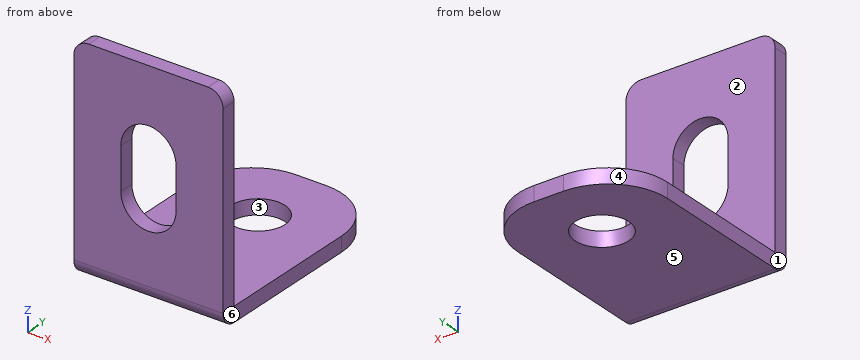
Autodesk Inventor part; units mm, degrees
ref_plane "YZ Plane" through (0, 0, 0) normal (1, 0, 0) x (0, 1, 0)
ref_plane "XZ Plane" through (0, 0, 0) normal (0, 1, 0) x (-1, 0, 0)
ref_plane "XY Plane" through (0, 0, 0) normal (0, 0, 1) x (1, 0, 0)
sketch "Sketch1" plane through (0, 0, 0) normal (0, 1, 0) x (-1, 0, 0)
  line L0 (5, 7.3) -> (-5, 7.3)
  line L1 (-5, 7.3) -> (-5, -7.3)
  line L2 (-5, -7.3) -> (5, -7.3)
  line L3 (5, -7.3) -> (5, 7.3)
  line L4 (5, 7.3) -> (-5, -7.3) construction
  line L5 (-5, 7.3) -> (5, -7.3) construction
  point P0 (0, 0)
  dimension "d0" = 10
  dimension "d1" = 14.6
extrude "Extrusion1" add sketch "Sketch1" along normal blind 1
sketch "Sketch2" plane through (5, 0, -7.3) normal (0, 0, -1) x (-1, 0, 0)
  line L0 (0, 0) -> (10, 0)
  line L1 (0, 0) -> (0, 14.7)
  line L2 (0, 14.7) -> (10, 14.7)
  line L3 (10, 14.7) -> (10, 0)
  point P0 (5, 0)
  dimension "d4" = 14.7
extrude "Extrusion2" add sketch "Sketch2" against normal blind 1
fillet "Fillet1" radius 4 2 edges at (5, 14.7, -6.8) (-5, 14.7, -6.8)
fillet "Fillet2" radius 1 2 edges at (-5, 0.5, 7.3) (5, 0.5, 7.3)
fillet "Fillet3" radius 1 1 edges at (0, 0, -7.3)
sketch "Sketch3" plane through (1, 14.7, -7.3) normal (0, 0, -1) x (-1, 0, 0)
  circle A0 centre (1, -4.8) radius 1.8
  line L0 (-4, -13.7) -> (-4, -4)
  line L1 (1, -3) -> (2.7418, -3) construction
  line L2 (2, 0) -> (0, 0) construction
  point P0 (1, -14.7)
  dimension "d12" = 3.6
  dimension "d10" = 5
  dimension "d11" = 3
extrude "Extrusion3" cut sketch "Sketch3" against normal blind 1
sketch "Sketch4" plane through (0, 0, 0) normal (0, -1, 0) x (1, 0, 0)
  line L0 (5, 6.3) -> (5, -6.3)
  line L1 (0, 3.6) -> (1.5693, 3.6) construction
  line L2 (-4, 7.3) -> (4, 7.3)
  line L3 (0, -2.9) -> (1.85, -2.9) construction
  line L4 (1.85, 1.75) -> (1.85, -1.05)
  line L5 (-1.85, 1.75) -> (-1.85, -1.05)
  arc A0 (1.85, 1.75) -> (-1.85, 1.75) centre (0, 1.75) ccw
  arc A1 (-1.85, -1.05) -> (1.85, -1.05) centre (0, -1.05) ccw
  line L6 (-5, -6.3) -> (-5, 6.3)
  point P0 (0, 0)
  dimension "d16" = 5
  dimension "d17" = 3.7
  dimension "d19" = 6.5
  dimension "d20" = 3.15
  dimension "d21" = 3.15
extrude "Extrusion4" cut sketch "Sketch4" against normal blind 1
properties part number "angle bracket short"
Build history of the part. All positions in model axes, mm. Face numbers are marked on the shaded views. A direction names the side the tool comes from. Give positions to 0.01 mm unless a question says otherwise; leave off trailing zeros. Order: outer loops, then holes, each group sorted by start corner. A loop starts at its lowest first (then second) coordinate and runs counter-clockwise, first axis right, second up. Notation, with made-up numbers: M 23.5,88.5 L 70.5,88.5 A21 ccw 70.5,120.5 Z; hole C 86,14.25 d7. An arc over 180 degrees is marked long. Return JSON: item names as keys, results as strings.
Q1. Wall check: probe 1 along Z at (x, y) = (2.5, 11); probe 2 along Y at (x, z) = (0, -6.5); probe 3 along Y at (x, z) = (-3.75, -1.5). Give the ranges that are in metal, low to high. Write a range as from..to.
Answer list:
{"probe 1": "z = -7.3..-6.3", "probe 2": "y = 0.02..8.1, 11.7..14.7", "probe 3": "y = 0..1"}
Q2. Band-saw the part on A-A (x = 0). Give the cut face in (y, z).
Answer list:
{"outline": "M 0,-6.3 A1 ccw 1,-7.3 L 8.1,-7.3 L 8.1,-6.3 L 1,-6.3 L 1,-2.9 L 0,-2.9 Z; M 0,3.6 L 1,3.6 L 1,7.3 L 0,7.3 Z; M 11.7,-7.3 L 14.7,-7.3 L 14.7,-6.3 L 11.7,-6.3 Z"}
Q3. Flat gauge pin, fed straight in: pin 1 (6 mm diameter, centred on x = 0, y = 7, fed in from +Z). Where does the tip first touch, or does it go through?
Answer list:
{"pin 1": "stops at z = -6.3"}
Q4. Band-saw the part on C-C (z = 1). Give the cut face in (x, y).
Answer list:
{"outline": "M -5,0 L -1.85,0 L -1.85,1 L -5,1 Z; M 1.85,0 L 5,0 L 5,1 L 1.85,1 Z"}
Q5. Band-saw the part on B-B (y = 9.9). Give the cut face in (x, z), then the cut area to 3 significant figures.
Answer list:
{"outline": "M -5,-7.3 L -1.8,-7.3 L -1.8,-6.3 L -5,-6.3 Z; M 1.8,-7.3 L 5,-7.3 L 5,-6.3 L 1.8,-6.3 Z", "area": "6.40 mm^2"}
Q6. Two-plate mould, pull along X, no slides. Class the marked faces 3, 4, 5 and 6: pulls with the +X half, pulls with the -X half, needs draft (parallel to the pull), parting line crosses it, or undercut.
Answer list:
{"face 3": "undercut", "face 4": "pulls with the -X half", "face 5": "needs draft", "face 6": "pulls with the +X half"}
Q7. 3-axis set-ups, long thin cutter, end or side, ignore diameter. For the marked faces 1 and 2: which of +Z, -Z, +X, -X, +Y, -Y reach the whole face in a straight line?
Answer list:
{"face 1": "+Z, -Z, -X, +Y, -Y", "face 2": "+Z, +X, -X, +Y"}
Q8. Band-saw the part on D-D (x = 1.5). Give the cut face in (y, z), then the cut area to 3 significant figures.
Answer list:
{"outline": "M 0,-6.3 A1 ccw 1,-7.3 L 8.91,-7.3 L 8.91,-6.3 L 1,-6.3 L 1,-2.13 L 0,-2.13 Z; M 0,2.83 L 1,2.83 L 1,7.3 L 0,7.3 Z; M 10.89,-7.3 L 14.67,-7.3 L 14.67,-6.3 L 10.89,-6.3 Z", "area": "21.1 mm^2"}
